```python
from build123d import *

# Parameters (mm, degrees)
F0_W     = 74.6
F0_H     = 50
F0_W_2   = 52.4393096566
F0_H_2   = 25.6734117866
F0_R     = 1.25
F1_DEPTH = 2
F2_DEPTH = 5
F3_DEPTH = 10
F4_R     = 3
F5_R     = 3


with BuildPart() as f1:
    # F0 (on Top) → F1 (new body)
    with BuildSketch(Plane.XY):
        Rectangle(F0_W, F0_H)
        with BuildLine():
            Line((-32.3, -20), (-32.3, 20))
            Line((-32.3, 20), (-31.0874586088, 20))
            ThreePointArc((-31.0874586088, 20), (-29.2, 20.75), (-27.3125413912, 20))
            Line((-27.3125413912, 20), (27.5244719095, 20))
            ThreePointArc((27.5244719095, 20), (29.3, 20.65), (31.0755280905, 20))
            Line((31.0755280905, 20), (32.3, 20))
            Line((32.3, 20), (32.3, -20))
            Line((32.3, -20), (31.0755280905, -20))
            ThreePointArc((31.0755280905, -20), (29.3, -20.65), (27.5244719095, -20))
            Line((27.5244719095, -20), (-27.3125413912, -20))
            ThreePointArc((-27.3125413912, -20), (-29.2, -20.75), (-31.0874586088, -20))
            Line((-31.0874586088, -20), (-32.3, -20))
        make_face(mode=Mode.SUBTRACT)
        with BuildLine():
            Line((-31.0874586088, 20), (-32.3, 20))
            Line((-32.3, 20), (-32.3, -20))
            Line((-32.3, -20), (-31.0874586088, -20))
            ThreePointArc((-31.0874586088, -20), (-30.289033706, -15.4748256323), (-26.45, -18))
            ThreePointArc((-26.45, -18), (-26.6748256323, -19.089033706), (-27.3125413912, -20))
            Line((-27.3125413912, -20), (27.5244719095, -20))
            ThreePointArc((27.5244719095, -20), (28.1424599896, -15.4054857939), (32.05, -17.9))
            ThreePointArc((32.05, -17.9), (31.7945142061, -19.0575400104), (31.0755280905, -20))
            Line((31.0755280905, -20), (32.3, -20))
            Line((32.3, -20), (32.3, 20))
            Line((32.3, 20), (31.0755280905, 20))
            ThreePointArc((31.0755280905, 20), (31.7945142061, 19.0575400104), (32.05, 17.9))
            ThreePointArc((32.05, 17.9), (28.1424599896, 15.4054857939), (27.5244719095, 20))
            Line((27.5244719095, 20), (-27.3125413912, 20))
            ThreePointArc((-27.3125413912, 20), (-26.6748256323, 19.089033706), (-26.45, 18))
            ThreePointArc((-26.45, 18), (-30.289033706, 15.4748256323), (-31.0874586088, 20))
        make_face()
        Rectangle(F0_W_2, F0_H_2, mode=Mode.SUBTRACT)
        with BuildLine():
            Line((31.0755280905, 20), (27.5244719095, 20))
            ThreePointArc((27.5244719095, 20), (28.1424599896, 15.4054857939), (32.05, 17.9))
            ThreePointArc((32.05, 17.9), (31.7945142061, 19.0575400104), (31.0755280905, 20))
        make_face()
        with Locations((29.3, 17.9)):
            Circle(F0_R, mode=Mode.SUBTRACT)
        with BuildLine():
            ThreePointArc((-26.45, -18), (-30.289033706, -15.4748256323), (-31.0874586088, -20))
            Line((-31.0874586088, -20), (-27.3125413912, -20))
            ThreePointArc((-27.3125413912, -20), (-26.6748256323, -19.089033706), (-26.45, -18))
        make_face()
        with Locations((-29.2, -18)):
            Circle(F0_R, mode=Mode.SUBTRACT)
        with Locations((-29.2, -18)):
            Circle(F0_R)
        with Locations((29.3, 17.9)):
            Circle(F0_R)
        with BuildLine():
            Line((-27.3125413912, -20), (-31.0874586088, -20))
            ThreePointArc((-31.0874586088, -20), (-29.2, -20.75), (-27.3125413912, -20))
        make_face()
    extrude(amount=F1_DEPTH)

    # F0 (on Top) → F2 (join)
    with BuildSketch(Plane.XY):
        with BuildLine():
            ThreePointArc((31.0755280905, 20), (29.3, 20.65), (27.5244719095, 20))
            Line((27.5244719095, 20), (31.0755280905, 20))
        make_face()
        with BuildLine():
            Line((31.0755280905, 20), (27.5244719095, 20))
            ThreePointArc((27.5244719095, 20), (28.1424599896, 15.4054857939), (32.05, 17.9))
            ThreePointArc((32.05, 17.9), (31.7945142061, 19.0575400104), (31.0755280905, 20))
        make_face()
        with Locations((29.3, 17.9)):
            Circle(F0_R, mode=Mode.SUBTRACT)
        with Locations((29.3, 17.9)):
            Circle(F0_R)
        with BuildLine():
            ThreePointArc((-26.45, -18), (-30.289033706, -15.4748256323), (-31.0874586088, -20))
            Line((-31.0874586088, -20), (-27.3125413912, -20))
            ThreePointArc((-27.3125413912, -20), (-26.6748256323, -19.089033706), (-26.45, -18))
        make_face()
        with Locations((-29.2, -18)):
            Circle(F0_R, mode=Mode.SUBTRACT)
        with Locations((-29.2, -18)):
            Circle(F0_R)
        with BuildLine():
            Line((-27.3125413912, -20), (-31.0874586088, -20))
            ThreePointArc((-31.0874586088, -20), (-29.2, -20.75), (-27.3125413912, -20))
        make_face()
        with BuildLine():
            Line((-27.3125413912, 20), (-31.0874586088, 20))
            ThreePointArc((-31.0874586088, 20), (-30.289033706, 15.4748256323), (-26.45, 18))
            ThreePointArc((-26.45, 18), (-26.6748256323, 19.089033706), (-27.3125413912, 20))
        make_face()
        with BuildLine():
            ThreePointArc((-27.3125413912, 20), (-29.2, 20.75), (-31.0874586088, 20))
            Line((-31.0874586088, 20), (-27.3125413912, 20))
        make_face()
        with BuildLine():
            ThreePointArc((32.05, -17.9), (28.1424599896, -15.4054857939), (27.5244719095, -20))
            Line((27.5244719095, -20), (31.0755280905, -20))
            ThreePointArc((31.0755280905, -20), (31.7945142061, -19.0575400104), (32.05, -17.9))
        make_face()
        with BuildLine():
            Line((31.0755280905, -20), (27.5244719095, -20))
            ThreePointArc((27.5244719095, -20), (29.3, -20.65), (31.0755280905, -20))
        make_face()
    extrude(amount=F2_DEPTH)

    # F0 (on Top) → F3 (join)
    with BuildSketch(Plane.XY):
        with Locations((29.3, 17.9)):
            Circle(F0_R)
        with Locations((-29.2, -18)):
            Circle(F0_R)
    extrude(amount=F3_DEPTH)

    # F4
    f4_edges = [f1.edges().sort_by_distance(p)[0] for p in [
        (37.3, 25, 1),
        (37.3, -25, 1),
        (-37.3, -25, 1),
        (-37.3, 25, 1),
    ]]
    fillet(f4_edges, radius=F4_R)

    # F5
    f5_edges = [f1.edges().sort_by_distance(p)[0] for p in [
        (-26.219655, 12.836706, 1),
        (26.219655, 12.836706, 1),
        (26.219655, -12.836706, 1),
        (-26.219655, -12.836706, 1),
    ]]
    fillet(f5_edges, radius=F5_R)


solid = f1.part
```
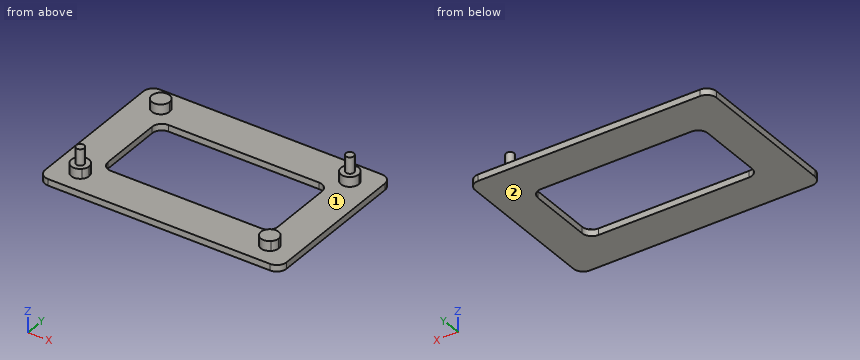
Model file for the job. Use its own axes, mm. Face numbers are marked on the shaded views. Round coordinates to 2 decimals unless told otherwise and drop trailing zeros. Write each loop counter-clockwise with the first axis right and the second up, starting at its lowest first coordinate (ties: lowest second). Pieces come first, ordered by that corner, then holes. Notation, with made-up numbers: (12, -3.75) -> (71, -3.75) arc R28 cw to (71, 18.25) -> close; hole circle Ø11 at (83, 70). An arc over 180 degrees is marked (long way). Answer as CSV lines item,"result".
1. Slice it at A-A, the plane y = 6.5. List the corners of the cut face in (x, z), plus the area to 3 significant figures.
Resolved:
outline,"(-37.3, 0) -> (-26.22, 0) -> (-26.22, 2) -> (-37.3, 2) -> close; (26.22, 0) -> (37.3, 0) -> (37.3, 2) -> (26.22, 2) -> close"
area,"44.3 mm²"
2. Pin check, flat tips, straight feed: pin 1 Ø5 at (x, z) = (-1.5, 6.5) entering from -Y; pin 2 Ø1.7 at (x, y) = (29, -17) entering from +Z. Stop position of each tip, or through.
Resolved:
pin 1,"through"
pin 2,"z = 5"
3. Slice it at B-B, the plane z = 3.5. List the corners of the cut face in (x, y).
Resolved:
outline,"circle Ø5.5 at (-29.2, -18); circle Ø5.5 at (-29.2, 18); circle Ø5.5 at (29.3, -17.9); circle Ø5.5 at (29.3, 17.9)"
4. Slice it at D-D, the plane x = 29.3. List the corners of the cut face in (y, z).
Resolved:
outline,"(-25, 0) -> (25, 0) -> (25, 2) -> (20.65, 2) -> (20.65, 5) -> (19.15, 5) -> (19.15, 10) -> (16.65, 10) -> (16.65, 5) -> (15.15, 5) -> (15.15, 2) -> (-15.15, 2) -> (-15.15, 5) -> (-20.65, 5) -> (-20.65, 2) -> (-25, 2) -> close"
5. Slice it at C-C, the plane x = -0.5. List the corners of the cut face in (y, z).
Resolved:
outline,"(-25, 0) -> (-12.84, 0) -> (-12.84, 2) -> (-25, 2) -> close; (12.84, 0) -> (25, 0) -> (25, 2) -> (12.84, 2) -> close"
6. Drill centre lines: line 1 (Y direction, x = -13, z = 0.5); line 2 (X direction, y = 6.5, z = 1); line 3 (Z direction, x = -3.5, y = 18.5). Where is each one in solid material? Low to high.
Resolved:
line 1,"-25 to -12.84, 12.84 to 25"
line 2,"-37.3 to -26.22, 26.22 to 37.3"
line 3,"0 to 2"
7. Mould opens along X. For the marked faces 1 and 2 say: +X half, -X half, draft (parallel to the pull), parting line (faces both ways), or undercut.
Resolved:
face 1,"undercut"
face 2,"draft"
